```python
from build123d import *

# Parameters (mm, degrees)
SKETCH1_W           = 50.8
SKETCH1_H           = 25.4
SKETCH1_W_2         = 47.625
SKETCH1_H_2         = 22.225
BOSS_EXTRUDE1_DEPTH = 304.8
SKETCH3_R           = 8.346891379
SKETCH3_R_2         = 3.175
SKETCH3_R_3         = 1.5875
SKETCH3_W           = 25.4
SKETCH3_H           = 50.8
CUT_EXTRUDE2_DEPTH  = 25.4


with BuildPart() as part:
    # Sketch1 → Boss-Extrude1 (new body)
    with BuildSketch(Plane.XY):
        Rectangle(SKETCH1_W, SKETCH1_H)
        Rectangle(SKETCH1_W_2, SKETCH1_H_2, mode=Mode.SUBTRACT)
    extrude(amount=BOSS_EXTRUDE1_DEPTH)

    # Sketch3 → Cut-Extrude2 (cut)
    with BuildSketch(Plane(origin=(0, 12.7, 0), x_dir=(1, 0, 0), z_dir=(0, 1, 0))):
        with Locations((0, -283.999565344)):
            Circle(SKETCH3_R)
        with Locations((0, -235.857473267)):
            Circle(SKETCH3_R_2)
        with Locations((-12.7, -248.557473267)):
            Circle(SKETCH3_R_3)
        with Locations((12.7, -223.157473267)):
            Circle(SKETCH3_R_3)
        with Locations((0, -183.469973267)):
            Rectangle(SKETCH3_W, SKETCH3_H)
        with Locations((0, -119.969973267)):
            Rectangle(SKETCH3_W, SKETCH3_H)
        with Locations((0, -56.469973267)):
            Rectangle(SKETCH3_W, SKETCH3_H)
    extrude(amount=-CUT_EXTRUDE2_DEPTH, mode=Mode.SUBTRACT)


solid = part.part
```
Geometry: final body of the model. Coordinates: model frame, mm. A direction names the side the tool comes from. Coordinates: 2 decimals unless noted, no trailing zeros. Order: outer loops, then holes, each group sorted by start corner. A loop starts at its lowest first (then second) coordinate and runs counter-clockwise, first axis right, second up. Notation, with made-up numbers: (88.5, 6.5) - (145.5, 6.5) arc R8 ccw to (145.5, 11.5) - close; hole circle Ø6 at (19, -10.5). An arc over 180 degrees is marked (long way). Write each question's results on one line, items separated by ' | '.
1) Section B-B, the plane y = 5.25. Return loops of the section in (x, z).
Results list:
outline: (-25.4, 0) - (-23.81, 0) - (-23.81, 304.8) - (-25.4, 304.8) - close; (23.81, 0) - (25.4, 0) - (25.4, 304.8) - (23.81, 304.8) - close
2) Section C-C, the plane z = 178. Return loops of the section in (x, y).
Results list:
outline: (-25.4, -12.7) - (-12.7, -12.7) - (-12.7, -11.11) - (-23.81, -11.11) - (-23.81, 11.11) - (-12.7, 11.11) - (-12.7, 12.7) - (-25.4, 12.7) - close; (12.7, -12.7) - (25.4, -12.7) - (25.4, 12.7) - (12.7, 12.7) - (12.7, 11.11) - (23.81, 11.11) - (23.81, -11.11) - (12.7, -11.11) - close
3) Pin query (flat end, axial travel): pin 1 (0.5 mm diameter, centred on x = 4.5, y = -12, fed in from -Z). Return the tip coordinate at first contact, or that it passes through.
Results list:
pin 1: z = 0
4) Pull-direction query (X, two-part tool) for faces 3 (the flat face through (0, -11.112, 150)), 4 (the flat face through (0, 12.7, 150)), 5 (the flat face through (25.4, 0, 150)); classes: pulls with the +X half, pulls with the -X half, needs draft (parallel to the pull), parting line crosses it, or undercut.
Results list:
face 3: undercut | face 4: needs draft | face 5: pulls with the +X half
5) Section D-D, the plane x = 0. State how many separate pieces and enclosed holes the cut face has, plus the area to 3 significant figures.
Results list:
separate pieces: 12 | enclosed holes: 0 | area: 411 mm^2
6) Section A-A, the plane x = 20. Return loops of the section in (y, z), plus the area to 3 significant figures.
Results list:
outline: (-12.7, 0) - (-11.11, 0) - (-11.11, 304.8) - (-12.7, 304.8) - close; (11.11, 0) - (12.7, 0) - (12.7, 304.8) - (11.11, 304.8) - close | area: 968 mm^2
7) Set-up query: faces 1 (the flat face through (0, -12.7, 150)), 2 (the flat face through (23.812, 0, 150)). Return all of +Z, -Z, +X, -X, +Y, -Y with unobstructed straight access to the full face (end or side cutting, diameter ignored); none if empty.
Results list:
face 1: +Z, -Z, +X, -X, -Y | face 2: +Z, -Z
8) Line query: line 1 (X direction, y = 8.5, z = 199); line 2 (Y direction, x = 21, z = 60). Output: solid intervals per line, ascending. Write a range as from..to.
Results list:
line 1: -25.4..-23.81, 23.81..25.4 | line 2: -12.7..-11.11, 11.11..12.7
